Autodesk Inventor part; units mm, degrees
ref_plane "YZ Plane" through (0, 0, 0) normal (1, 0, 0) x (0, 1, 0)
ref_plane "XZ Plane" through (0, 0, 0) normal (0, 1, 0) x (-1, 0, 0)
ref_plane "XY Plane" through (0, 0, 0) normal (0, 0, 1) x (1, 0, 0)
sketch "Sketch1" plane through (0, 0, 0) normal (1, 0, 0) x (0, 1, 0)
  circle A0 centre (0, 0) radius 17.4625
extrude "Extrusion1" add sketch "Sketch1" along normal blind 1.27
sketch "Sketch2" plane through (1.27, 0, 0) normal (1, 0, 0) x (0, 0, -1)
  circle A0 centre (0, 15.168) radius 1.27
  circle A1 centre (0, -14.7346) radius 1.27
  point P0 (0, 0)
extrude "Extrusion2" add sketch "Sketch2" along normal blind 88.9
sketch "Sketch3" plane through (90.17, 15.168, 0) normal (1, 0, 0) x (0, 0, -1)
  circle A0 centre (0, -15.168) radius 17.4625
extrude "Extrusion3" add sketch "Sketch3" against normal blind 82.55
sketch "Sketch4" plane through (1.27, 0, 0) normal (1, 0, 0) x (0, 0, -1)
  point P0 (0, 0)
sketch "Sketch5" plane through (1.27, 0, 0) normal (1, 0, 0) x (0, 0, -1)
  point P0 (0, 0)
extrude "Extrusion4" [suppressed]
properties part number "STACK NEW." material "Glass"
Input: part model. Units: mm. Frame: model coordinates. A direction names the side the tool comes from. Coordinates: 2 decimals unless noted, no trailing zeros. Loops run counter-clockwise (first coordinate to the right, second up) from the corner with the lowest first, then second, coordinate; pieces in that order, holes last. Notation, with made-up numbers: M 68,40.5 L 98,40.5 A16 ccw 98,64.5 Z; hole C 87.5,-11 d2. An arc over 180 degrees is marked long. Use a Markdown table: item, result. Add a question column.
1) Draft query along X for faces 1 (the cylindrical face through (4.401, -15.994, 0.165)), 2 (the flat face through (0, 0, 0)), 3 (the flat face through (90.17, 0, 0)). Return one class per face: +X half, -X half, draft (parallel to the pull), parting line (faces both ways), or undercut.
2) Section A-A, the plane y = 0. Return the cut outline in (x, z), plus the area to 3 significant figures.
3) Line query: L1, parallel to X at y = 14, z = -10; L2, parallel to Z at x = 37.5, y = -0.5; L3, parallel to Y at x = 8.5, z = -9. Output: solid intervals per line, ascending. Write a range as from..to.
4) Section D-D, the plane x = 13.5. Return the cut outline in (y, z) (1 decimal), plus the area to 3 significant figures.
5) Section C-C, the plane z = 0. Return the cut outline in (x, y), plus the area to 3 significant figures.
6) Section B-B, the plane z = 9. Return the cut outline in (x, y), plus the area to 3 significant figures.
7) Pin query (flat end, axial travel): P1, Ø6, axis at x = 55, y = 7.5, coming from the +Z side; P2, Ø4, axis at x = 69.5, y = 13, coming from the +Z side; P3, Ø2, axis at x = 57.5, y = 13, coming from the +Z side. Return the tip coordinate at first contact, or that it passes through.
8) Set-up query: faces 4 (the cylindrical face through (4.401, 16.408, 0.275)), 5 (the cylindrical face through (49.473, -10.626, 13.858)). Return all of +Z, -Z, +X, -X, +Y, -Y with unobstructed straight access to the full face (end or side cutting, diameter ignored); none if empty.
Answer below:
| question | item | result |
|---|---|---|
| 1 | face 1 | undercut |
| 1 | face 2 | -X half |
| 1 | face 3 | +X half |
| 2 | outline | M 0,-17.46 L 1.27,-17.46 L 1.27,17.46 L 0,17.46 Z; M 7.62,-17.46 L 90.17,-17.46 L 90.17,17.46 L 7.62,17.46 Z |
| 2 | area | 2,930 mm2 |
| 3 | L1 | 0..1.27, 7.62..90.17 |
| 3 | L2 | -17.46..17.46 |
| 3 | L3 | -14.96..14.96 |
| 4 | outline | C 0,0 d34.9 |
| 4 | area | 958 mm2 |
| 5 | outline | M 0,-17.46 L 1.27,-17.46 L 1.27,-16 L 7.62,-16 L 7.62,-17.46 L 90.17,-17.46 L 90.17,17.46 L 7.62,17.46 L 7.62,16.44 L 1.27,16.44 L 1.27,17.46 L 0,17.46 Z; hole M 1.27,-13.46 L 7.62,-13.46 L 7.62,13.9 L 1.27,13.9 Z |
| 5 | area | 2,960 mm2 |
| 6 | outline | M 0,-14.96 L 1.27,-14.96 L 1.27,14.96 L 0,14.96 Z; M 7.62,-14.96 L 90.17,-14.96 L 90.17,14.96 L 7.62,14.96 Z |
| 6 | area | 2,510 mm2 |
| 7 | P1 | z = 16.87 |
| 7 | P2 | z = 13.56 |
| 7 | P3 | z = 12.69 |
| 8 | face 4 | none |
| 8 | face 5 | +X, -X |
